Read the model definition and answer for the solid it produces. Units are mm, in the model's axes. Give positions to 0.01 mm unless a question says otherwise; leave off trailing zeros. Order: outer loops, then holes, each group sorted by start corner. A loop starts at its lowest first (then second) coordinate and runs counter-clockwise, first axis right, second up. Notation, with made-up numbers: (69.5, 77) - (91.5, 77) arc R15 ccw to (91.5, 84) - close; hole circle Ø11 at (74.5, 82.5). An arc over 180 degrees is marked (long way). One line per item, written item: value. Start each with the question number.
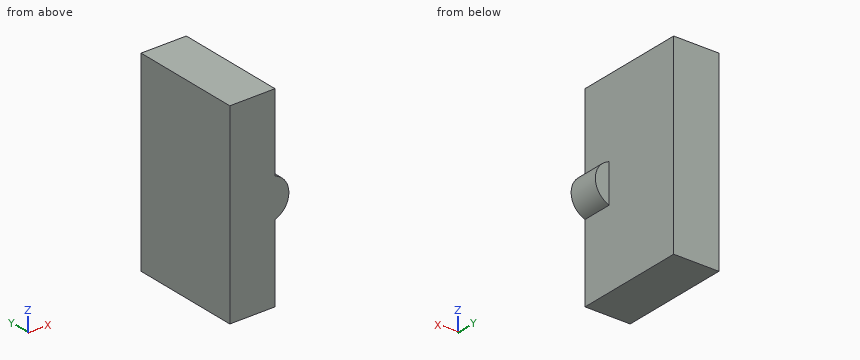
```python
from build123d import *

# Parameters (mm, degrees)
SKETCH1_R                = 31.5
BOSS_EXTRUDE1_DEPTH      = 170
SKETCH2_W                = 70
SKETCH2_H                = 300
BOSS_EXTRUDE2_DEPTH      = 125
BOSS_EXTRUDE2_DEPTH_BACK = 130
SKETCH2_2_W              = 70
SKETCH2_2_H              = 300
BOSS_EXTRUDE3_DEPTH      = 10
SKETCH4_W                = 315.689390272
SKETCH4_H                = 433.788608214
CUT_EXTRUDE2_DEPTH       = 123


with BuildPart() as part:
    # Sketch1 → Boss-Extrude1 (new body)
    with BuildSketch(Plane(origin=(0, 0, 0), x_dir=(1, 0, 0), z_dir=(0, 1, 0))):
        Circle(SKETCH1_R)
    extrude(amount=BOSS_EXTRUDE1_DEPTH)

    # Sketch2 → Boss-Extrude2 (add, two sides)
    with BuildSketch(Plane(origin=(0, 170, 0), x_dir=(1, 0, 0), z_dir=(0, 1, 0))) as boss_extrude2_sk:
        with Locations((-25, 0)):
            Rectangle(SKETCH2_W, SKETCH2_H)
    extrude(amount=BOSS_EXTRUDE2_DEPTH)
    extrude(boss_extrude2_sk.sketch, amount=-BOSS_EXTRUDE2_DEPTH_BACK)

    # Sketch2_2 → Boss-Extrude3 (add)
    with BuildSketch(Plane(origin=(0, 170, 0), x_dir=(1, 0, 0), z_dir=(0, 1, 0))):
        with Locations((-25, 0)):
            Rectangle(SKETCH2_2_W, SKETCH2_2_H)
    extrude(amount=BOSS_EXTRUDE3_DEPTH)

    # Sketch4 → Cut-Extrude2 (cut)
    with BuildSketch(Plane.XZ):
        Rectangle(SKETCH4_W, SKETCH4_H)
    extrude(amount=-CUT_EXTRUDE2_DEPTH, mode=Mode.SUBTRACT)


solid = part.part
```
1) Each of these flat-tipped pins is pushed along its axis until it touches: pin 1 (6.5 mm diameter, centred on x = 16, z = 1.5, fed in from +Y); pin 2 (1.5 mm diameter, centred on y = 216.5, z = -30.5, fed in from +X). Where does it stop, or does it pass through?
2) Section C-C on x = 22.5 is taken. Write down the section's boundary in (y, z), plus the area to 3 significant figures.
3) Section A-A on y = 139 is taken. Write down the section's boundary in (x, z).
4) Section B-B on z = 129 is taken. Write down the section's boundary in (x, y).
5) Find the intervals of material crossed by probe 1 along X at (y, z) = (270, -22); probe 2 along Z at (x, y) = (15, 163); probe 3 along Z at (x, y) = (22.5, 157), in increasing order. Write a range as from..to.
Solved:
1. pin 1: stops at y = 170
1. pin 2: stops at x = 10
2. outline: (123, -22.05) - (170, -22.05) - (170, 22.05) - (123, 22.05) - close
2. area: 2,070 mm2
3. outline: (-60, -150) - (10, -150) - (10, -29.87) arc R31.5 ccw to (10, 29.87) - (10, 150) - (-60, 150) - close
4. outline: (-60, 123) - (10, 123) - (10, 295) - (-60, 295) - close
5. probe 1: x = -60..10
5. probe 2: z = -27.7..27.7
5. probe 3: z = -22.05..22.05
